The listing builds one solid part. Answer for the finished solid, in the listing's coordinates (mm). A direction names the side the tool comes from. Coordinates: 2 decimals unless noted, no trailing zeros. Order: outer loops, then holes, each group sorted by start corner. A loop starts at its lowest first (then second) coordinate and runs counter-clockwise, first axis right, second up.
from build123d import *

# Parameters (mm, degrees)
F3_DEPTH = 4
F4_SIZE  = 1


with BuildPart() as f1:
    # F0 (on Front) → F1 (revolve)
    with BuildSketch(Plane.XZ):
        Polygon((-17.0283879898, 10.2372211188), (-17.0283879898, 15.9372211188), (-27.0283879898, 15.9372211188), (-27.0283879898, 13.9372211188), (-22.4783879898, 13.9372211188), (-22.4783879898, 13.2372211188), (-20.9783879898, 13.2372211188), (-20.9783879898, 10.5372211188), (-21.1783879898, 10.5372211188), (-21.1783879898, 10.2372211188), align=None)
    revolve(axis=Axis((-17.0283879898, 0, 13.0872211188), (0, 0, -1)))

    # F2 (on face) → F3 (cut)
    with BuildSketch(Plane(origin=(0, 0, 10.2372211188), x_dir=(1, 0, 0), z_dir=(0, 0, -1))):
        with BuildLine():
            Line((-21.1481574009, -0.5), (-18.705438973, -0.5))
            ThreePointArc((-18.705438973, -0.5), (-17.0283879898, -1.75), (-15.3513370067, -0.5))
            Line((-15.3513370067, -0.5), (-12.9086185788, -0.5))
            ThreePointArc((-12.9086185788, -0.5), (-12.8859525313, -0.2504565274), (-12.8783879898, 0))
            ThreePointArc((-12.8783879898, 0), (-12.8859525313, 0.2504565274), (-12.9086185788, 0.5))
            Line((-12.9086185788, 0.5), (-15.3513370067, 0.5))
            ThreePointArc((-15.3513370067, 0.5), (-17.0283879898, 1.75), (-18.705438973, 0.5))
            Line((-18.705438973, 0.5), (-21.1481574009, 0.5))
            ThreePointArc((-21.1481574009, 0.5), (-21.1783879898, 0), (-21.1481574009, -0.5))
        make_face()
    extrude(amount=-F3_DEPTH, mode=Mode.SUBTRACT)

    # F4
    f4_edges = [f1.edges().sort_by_distance(p)[0] for p in [
        (-7.028388, 0, 15.937221),
    ]]
    chamfer(f4_edges, length=F4_SIZE)


solid = f1.part
(1) Find the intervals of material crossed by probe 1 along Z at (x, y) = (-9.25, -1.5); probe 2 along X at (y, z) = (-1.25, 12.45); probe 3 along Y at (x, z) = (-15, 12.15), in increasing order.
(2) Given pin 1 Ø1.5 at (y, z) = (3, 11) entering from -X; pin 2 Ø1 at (y, z) = (2.5, 12.5) entering from +X; pin 3 Ø0.7 at (x, z) = (-14, 11.5) entering from -Y, each flat-ended and moving along its own axis, determine where each tip first touches the part or whether it passes through.
(3) Find section B-B on z = 15.5. Determine the outline of the cut face in (x, y), then the cut area to 3 significant figures.
(4) A tool of negligible diameter and unlimited length cuts with its end or side. For faces 4 (the cylindrical face through (-17, -1.75, 12.21)), 5 (the flat face through (-17, -2, 10.237)), from which of +Z, -Z, +X, -X, +Y, -Y can it reach the whole face along a straight path? Write none if from no direction.
(5) Find section A-A on z = 11.8. Determine the outline of the cut face in (x, y).
(6) The mould has two halves that part along Z. Classify faces 1 (the cylindrical face through (-16.95, -3.95, 11.87)), 2 (the flat face through (-21, -4, 13.937)), 3 (the flat face through (-20, 0.5, 12)): pulls with the +Z half, pulls with the -Z half, needs draft (parallel to the pull), parting line crosses it, or undercut.
Resolved:
1. probe 1: z = 13.94 to 15.94
1. probe 2: x = -20.78 to -18.25, -15.8 to -13.28
1. probe 3: y = -3.39 to -0.5, 0.5 to 3.39
2. pin 1: stops at x = -20.41
2. pin 2: stops at x = -13.62
2. pin 3: stops at y = -2.9
3. outline: circle Ø18.87 at (-17.03, 0)
3. area: 280 mm2
4. face 4: -Z
4. face 5: -Z, +X, -X, +Y, -Y
5. outline: (-20.95, -0.5) arc R3.95 ccw to (-13.11, -0.5) - (-15.35, -0.5) arc R1.75 cw to (-18.71, -0.5) - close; (-20.95, 0.5) - (-18.71, 0.5) arc R1.75 cw to (-15.35, 0.5) - (-13.11, 0.5) arc R3.95 ccw to start
6. face 1: undercut
6. face 2: pulls with the -Z half
6. face 3: needs draft
